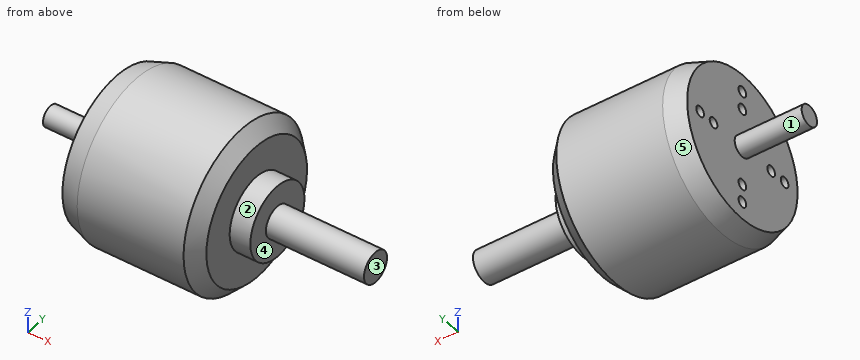
```python
from build123d import *

# Parameters (mm, degrees)
SKETCH2_R           = 4
BOSS_EXTRUDE1_DEPTH = 26
SKETCH3_R           = 31.3
BOSS_EXTRUDE2_DEPTH = 54
SKETCH4_R           = 2
CUT_EXTRUDE1_DEPTH  = 8
CHAMFER1_SIZE       = 2.54
CHAMFER1_SIZE2      = 7.62
CHAMFER2_SIZE       = 5.08
SKETCH5_R           = 14.097
BOSS_EXTRUDE3_DEPTH = 8.0264
SKETCH6_R           = 5.9944
BOSS_EXTRUDE4_DEPTH = 38.1


with BuildPart() as part:
    # Sketch2 → Boss-Extrude1 (new body)
    with BuildSketch(Plane(origin=(0, 0, 0), x_dir=(0, 0, -1), z_dir=(1, 0, 0))):
        Circle(SKETCH2_R)
    extrude(amount=BOSS_EXTRUDE1_DEPTH)

    # Sketch3 → Boss-Extrude2 (add)
    with BuildSketch(Plane(origin=(26, 0, 0), x_dir=(0, 0, -1), z_dir=(1, 0, 0))):
        Circle(SKETCH3_R)
    extrude(amount=BOSS_EXTRUDE2_DEPTH)

    # Sketch4 → Cut-Extrude1 (cut)
    with BuildSketch(Plane.ZY.offset(-26)):
        with Locations((15, 0)):
            Circle(SKETCH4_R)
        with Locations((0, -22)):
            Circle(SKETCH4_R)
        with Locations((0, -15)):
            Circle(SKETCH4_R)
        with Locations((-15, 0)):
            Circle(SKETCH4_R)
        with Locations((0, 15)):
            Circle(SKETCH4_R)
        with Locations((0, 22)):
            Circle(SKETCH4_R)
        with Locations((22, 0)):
            Circle(SKETCH4_R)
        with Locations((-22, 0)):
            Circle(SKETCH4_R)
    extrude(amount=-CUT_EXTRUDE1_DEPTH, mode=Mode.SUBTRACT)

    # Chamfer1
    chamfer1_edges = [part.edges().sort_by_distance(p)[0] for p in [
        (26, 0, 31.3),
    ]]
    chamfer1_side = [part.faces().sort_by_distance(p)[0] for p in [
        (26, 0, 30.41470231),
    ]]
    chamfer(chamfer1_edges, length=CHAMFER1_SIZE, length2=CHAMFER1_SIZE2, reference=chamfer1_side[0])

    # Chamfer2
    chamfer2_edges = [part.edges().sort_by_distance(p)[0] for p in [
        (80, 0, 31.3),
    ]]
    chamfer(chamfer2_edges, length=CHAMFER2_SIZE)

    # Sketch5 → Boss-Extrude3 (add)
    with BuildSketch(Plane(origin=(80, 0, 0), x_dir=(0, 0, -1), z_dir=(1, 0, 0))):
        Circle(SKETCH5_R)
    extrude(amount=BOSS_EXTRUDE3_DEPTH)

    # Sketch6 → Boss-Extrude4 (add)
    with BuildSketch(Plane(origin=(88.0264, 0, 0), x_dir=(0, 0, -1), z_dir=(1, 0, 0))):
        Circle(SKETCH6_R)
    extrude(amount=BOSS_EXTRUDE4_DEPTH)


solid = part.part
```
The model under review builds one solid part; all positions refer to its coordinate system, in mm. Face numbers are marked on the shaded views. A direction names the side the tool comes from. Give positions to 0.01 mm unless a question says otherwise; leave off trailing zeros. Write each loop counter-clockwise with the first axis right and the second up, starting at its lowest first coordinate (ties: lowest second). Pieces come first, ordered by that corner, then holes.
(1) Consider section A-A, the plane x = 65. Give the boundary of the cut face in (y, z).
(2) To check wall thickness, follow L1, parallel to X at y = 13, z = -21.5; L2, parallel to Y at x = 31, z = 0; L3, parallel to Y at x = 29.75, z = 15. State the ranges of each line that lie inside material, in increasing order.
(3) For P1, Ø2.5, axis at y = 15, z = 0, coming from the -X side; P2, Ø8, axis at x = 43.5, z = -1.5, coming from the +Y side; P3, Ø2, axis at y = 0.5, z = 16, coming from the -X side, all flat-tipped, find the tip position at first contact; note any pin that passes through.
(4) Tool access review of the marked faces 1, 2 and 3: name each direction out of +Z, -Z, +X, -X, +Y, -Y from which nothing blocks a thin tool from reaching the whole face with its end or side.
(5) The part is to be moulded in two halves that separate along Y. For the marked faces 4 and 5, say which applies: released by +Y, released by -Y, zero draft, split by the parting line, or undercut.
Returned:
1. outline: circle Ø62.6 at (0, 0)
2. L1: x = 26 to 80
2. L2: y = -30.43 to -24, -20 to -17, -13 to 13, 17 to 20, 24 to 30.43
2. L3: y = -25.99 to -2, 2 to 25.99
3. P1: stops at x = 34
3. P2: stops at y = 31.3
3. P3: stops at x = 26
4. face 1: -X
4. face 2: +X
4. face 3: +Z, -Z, +X, +Y, -Y
5. face 4: zero draft
5. face 5: split by the parting line
